Design review of the part built by this model. Coordinates are the model's own, in mm. A direction names the side the tool comes from. Round coordinates to 2 decimals unless told otherwise and drop trailing zeros. Order: outer loops, then holes, each group sorted by start corner. A loop starts at its lowest first (then second) coordinate and runs counter-clockwise, first axis right, second up. Notation, with made-up numbers: (-18.75, 13) - (-0.75, 13) arc R19 cw to (-0.75, 39) - close; hole circle Ø3 at (43.25, -38). An arc over 180 degrees is marked (long way). Use CSV: the item, a comma, the result in double quotes.
from build123d import *

# Parameters (mm, degrees)
F1_DEPTH = 7


with BuildPart() as f1:
    # F0 (on Top) → F1 (new body)
    with BuildSketch(Plane.XY):
        with BuildLine():
            ThreePointArc((-33.1978872418, 24.7798599303), (-33.0834757558, 22.7654689427), (-31.8994224072, 21.131798625))
            ThreePointArc((-31.8994224072, 21.131798625), (-37.9491495245, 16.6100964199), (-41.6069738567, 10.002123192))
            ThreePointArc((-41.6069738567, 10.002123192), (-39.5495454522, 3.3265737687), (-34.5581807196, -1.5603731154))
            ThreePointArc((-34.5581807196, -1.5603731154), (-19.8946406078, -7.2187581256), (-4.3225614354, -9.3511464074))
            Line((-4.3225614354, -9.3511464074), (0, -13.1228696555))
            Line((0, -13.1228696555), (3.8392005954, -9.3511464074))
            ThreePointArc((3.8392005954, -9.3511464074), (19.4504731476, -7.5377401012), (33.8274911046, -1.1893837946))
            ThreePointArc((33.8274911046, -1.1893837946), (39.9482242909, 4.9505196785), (39.2068363726, 13.5883511975))
            ThreePointArc((39.2068363726, 13.5883511975), (35.8899105198, 17.6875243488), (31.477894634, 20.5753147602))
            ThreePointArc((31.477894634, 20.5753147602), (32.4658862333, 22.5633647209), (32.5908623636, 24.7798599303))
            ThreePointArc((32.5908623636, 24.7798599303), (30.8966861442, 23.8400043647), (29.1282963008, 23.0485759676))
            ThreePointArc((29.1282963008, 23.0485759676), (30.4199988214, 26.5567217253), (30.1176030189, 30.2828643471))
            ThreePointArc((30.1176030189, 30.2828643471), (25.7979668662, 27.1597634239), (21.0283678025, 24.7798599303))
            ThreePointArc((21.0283678025, 24.7798599303), (10.6169463492, 26.9919126813), (0, 27.747772634))
            ThreePointArc((0, 27.747772634), (-10.9014405907, 27.0972820622), (-21.5735584497, 24.7798599303))
            ThreePointArc((-21.5735584497, 24.7798599303), (-26.3855190932, 27.1382027062), (-30.7246260345, 30.2828643471))
            ThreePointArc((-30.7246260345, 30.2828643471), (-30.9978734662, 26.4100339617), (-29.0551744401, 23.0485759676))
            ThreePointArc((-29.0551744401, 23.0485759676), (-31.282323769, 23.5414279438), (-33.1978872418, 24.7798599303))
        make_face()
        with BuildLine():
            ThreePointArc((-25.9017664939, -1.8695309991), (-33.7503475703, 7.0579634382), (-29.0551744401, 17.9783906788))
            Line((-29.0551744401, 17.9783906788), (-28.0658695847, 17.0509181917))
            ThreePointArc((-28.0658695847, 17.0509181917), (-30.1557554553, 13.105925168), (-30.106311664, 8.6418297142))
            Line((-30.106311664, 8.6418297142), (-32.0849195123, 9.5693022013))
            ThreePointArc((-32.0849195123, 9.5693022013), (-31.2882621481, 5.3843879138), (-28.2513629645, 2.3968447931))
            ThreePointArc((-28.2513629645, 2.3968447931), (-19.7085629501, -1.3566931507), (-10.3820515797, -1.0657209205))
            Line((-10.3820515797, -1.0657209205), (-11.4950193092, -4.1572973132))
            Line((-11.4950193092, -4.1572973132), (-8.0942846835, -3.1061612535))
            Line((-8.0942846835, -3.1061612535), (-6.1156759039, -7.0633799769))
            ThreePointArc((-6.1156759039, -7.0633799769), (-16.2750356162, -5.4809865628), (-25.9017664939, -1.8695309991))
        make_face(mode=Mode.SUBTRACT)
        with BuildLine():
            ThreePointArc((-6.4248335548, 5.6120846421), (-18.2829236305, 3.6515341791), (-23.5521681607, 14.4539931789))
            Line((-23.5521681607, 14.4539931789), (-14.9885008577, 10.0330389105))
            Line((-14.9885008577, 10.0330389105), (-11.4866484755, 8.2252235565))
            Line((-11.4866484755, 8.2252235565), (-6.4248335548, 5.6120846421))
        make_face(mode=Mode.SUBTRACT)
        with BuildLine():
            ThreePointArc((0, -10.1549560204), (-3.4356645233, -5.608379356), (-4.4462243095, 0))
            ThreePointArc((-4.4462243095, 0), (-2.9338853411, 3.8058939588), (0, 6.6632204689))
            ThreePointArc((0, 6.6632204689), (2.5812160346, 3.5845194486), (4.395684693, 0))
            ThreePointArc((4.395684693, 0), (3.2653866019, -5.5395763131), (0, -10.1549560204))
        make_face(mode=Mode.SUBTRACT)
        with BuildLine():
            ThreePointArc((28.3863190562, 17.7928954363), (32.9046262681, 11.0282269807), (30.9214107692, 3.138822969))
            ThreePointArc((30.9214107692, 3.138822969), (19.4051476303, -4.6231903079), (5.7559781708, -7.187042851))
            Line((5.7559781708, -7.187042851), (7.9819131643, -2.9206669424))
            Line((7.9819131643, -2.9206669424), (10.9170274232, -4.4520307225))
            Line((10.9170274232, -4.4520307225), (10.0223543122, -1.6222046688))
            ThreePointArc((10.0223543122, -1.6222046688), (18.8690080758, -1.3476793334), (27.0260237157, 2.0876871422))
            ThreePointArc((27.0260237157, 2.0876871422), (30.3026103064, 5.1576516383), (31.4160622656, 9.5074707642))
            Line((31.4160622656, 9.5074707642), (29.1901286691, 8.6418297142))
            ThreePointArc((29.1901286691, 8.6418297142), (29.2288443333, 12.8169576264), (27.6443399489, 16.6799277067))
            Line((27.6443399489, 16.6799277067), (28.3863190562, 17.7928954363))
        make_face(mode=Mode.SUBTRACT)
        with BuildLine():
            Line((11.4866484755, 8.2252235565), (14.9885008577, 10.0330389105))
            Line((14.9885008577, 10.0330389105), (23.5521681607, 14.4539931789))
            ThreePointArc((23.5521681607, 14.4539931789), (18.2829236305, 3.6515341791), (6.4248335548, 5.6120846421))
            Line((6.4248335548, 5.6120846421), (11.4866484755, 8.2252235565))
        make_face(mode=Mode.SUBTRACT)
        with BuildLine():
            ThreePointArc((-16.8125312775, 16.618097201), (-24.2503546691, 20.26833819), (-29.24066782, 26.8821306527))
            ThreePointArc((-29.24066782, 26.8821306527), (-22.7740559507, 22.7868013128), (-15.6377311796, 20.0188308954))
            ThreePointArc((-15.6377311796, 20.0188308954), (-7.2427370511, 15.8566956525), (-1.4164794702, 8.5181659088))
            ThreePointArc((-1.4164794702, 8.5181659088), (-8.8622483515, 13.047612435), (-16.8125312775, 16.618097201))
        make_face(mode=Mode.SUBTRACT)
        with BuildLine():
            ThreePointArc((16.8125312775, 16.618097201), (8.8622483515, 13.047612435), (1.4164794702, 8.5181659088))
            ThreePointArc((1.4164794702, 8.5181659088), (7.2427370511, 15.8566956525), (15.6377311796, 20.0188308954))
            ThreePointArc((15.6377311796, 20.0188308954), (22.7740559507, 22.7868013128), (29.24066782, 26.8821306527))
            ThreePointArc((29.24066782, 26.8821306527), (24.2503546691, 20.26833819), (16.8125312775, 16.618097201))
        make_face(mode=Mode.SUBTRACT)
    extrude(amount=F1_DEPTH)


solid = f1.part
1) For faces 1 (the face through (-31.317, 5.438, 3.451)), 2 (the face through (-39.6, 3.41, 3.45)), 3 (the face through (25.862, 27.199, 3.451)), list the 3-axis set-ups (+Z, -Z, +X, -X, +Y, -Y) from which the entire face can be reached by the end or side of a thin tool; tool diameter is ignored.
Data:
face 1,"+Z, -Z"
face 2,"+Z, -Z, -X, -Y"
face 3,"+Z, -Z, +Y"
2) We need section D-D (z = 1.5). Give the number of separate pieces and of enclosed holes in the cut face, then the cut area to 3 significant figures.
Data:
separate pieces,"1"
enclosed holes,"7"
area,"1,790 mm2"
3) Insertion check: pin 1 Ø1 at (x, z) = (25.5, 1.5) entering from -Y; pin 2 Ø3 at (y, z) = (-0.5, 4) entering from -X; pin 3 Ø1.5 at (x, z) = (-33, 4.5) entering from +Y. Each pin has a flat end and moves straight along its axis. Give the tip position at first contact, or say it passes through.
Data:
pin 1,"stops at y = -5.69"
pin 2,"stops at x = -37.78"
pin 3,"stops at y = 24.78"
4) To check wall thickness, follow L1, parallel to Y at x = -15.5, z = 4; L2, parallel to Y at x = 18, z = 2; L3, parallel to Y at x = 27.5, z = 4.5. State the ranges of each line that lie inside material, in increasing order. Write a range as from..to.
Data:
L1,"y = -8.2..-5.68, -1.74..2.7, 10.3..16.11, 19.98..26.31"
L2,"y = -7.91..-5.16, -1.52..3.51, 11.59..16.93, 20.76..25.58"
L3,"y = -4.62..0.08, 2.35..23.78, 25.6..28.26"
5) We need section C-C (y = 24). Give the boundary of the cut face in (x, z), then the cut area to 3 significant figures.
Data:
outline,"(-33.29, 0) - (-32.18, 0) - (-32.18, 7) - (-33.29, 7) - close; (-29.9, 0) - (-27.65, 0) - (-27.65, 7) - (-29.9, 7) - close; (-25, 0) - (25, 0) - (25, 7) - (-25, 7) - close; (27.65, 0) - (29.66, 0) - (29.66, 7) - (27.65, 7) - close; (31.21, 0) - (32.65, 0) - (32.65, 7) - (31.21, 7) - close"
area,"398 mm2"
6) We need section A-A (y = 1). Give the boundary of the cut face in (x, z), then the cut area to 3 significant figures.
Data:
outline,"(-37.78, 0) - (-30.69, 0) - (-30.69, 7) - (-37.78, 7) - close; (-26.1, 0) - (-4.22, 0) - (-4.22, 7) - (-26.1, 7) - close; (3.99, 0) - (25.21, 0) - (25.21, 7) - (3.99, 7) - close; (28.63, 0) - (37.36, 0) - (37.36, 7) - (28.63, 7) - close"
area,"412 mm2"
7) We need section B-B (x = -19). Give the boundary of the cut face in (y, z), then the cut area to 3 significant figures.
Data:
outline,"(-7.44, 0) - (-4.68, 0) - (-4.68, 7) - (-7.44, 7) - close; (-1.48, 0) - (4.06, 0) - (4.06, 7) - (-1.48, 7) - close; (12.1, 0) - (17.26, 0) - (17.26, 7) - (12.1, 7) - close; (21.12, 0) - (25.5, 0) - (25.5, 7) - (21.12, 7) - close"
area,"125 mm2"
